Verification items for the finished model (mm, model axes). Face numbers are marked on the shaded views. Give positions to 0.01 mm unless a question says otherwise; leave off trailing zeros. Loops run counter-clockwise (first coordinate to the right, second up) from the corner with the lowest first, then second, coordinate; pieces in that order, holes last. Notation, with made-up numbers: (23, 12) - (70, 12) arc R28 cw to (70, 49) - close; hole circle Ø1 at (52, 66). An arc over 180 degrees is marked (long way). Use one line per item in the form item = value.
```python
from build123d import *

# Parameters (mm, degrees)
SKETCH_1_W      = 134
SKETCH_1_H      = 90
EXTRUDE_1_DEPTH = 5
EXTRUDE_2_DEPTH = 10
EXTRUDE_3_DEPTH = 8


with BuildPart() as part:
    # Эскиз1 → Бобышка-Вытянуть1 (new body)
    with BuildSketch(Plane(origin=(0, 0, 0), x_dir=(1, 0, 0), z_dir=(0, 1, 0))):
        Rectangle(SKETCH_1_W, SKETCH_1_H)
    extrude(amount=EXTRUDE_1_DEPTH)

    # Эскиз2 → Бобышка-Вытянуть2 (add)
    with BuildSketch(Plane(origin=(0, 5, 0), x_dir=(1, 0, 0), z_dir=(0, 1, 0))):
        Polygon((-51.5, -45), (-47, -45), (-47, -25), (-52, -25), (-52, 30), (52, 30), (52, -25), (42, -25), (42, -45), (51.5, -45), (67, -45), (67, -25), (67, 30), (67, 45), (51.5, 45), (-51.5, 45), (-67, 45), (-67, 30), (-67, -25), (-67, -45), align=None)
    extrude(amount=EXTRUDE_2_DEPTH)

    # Эскиз3 → Бобышка-Вытянуть3 (add)
    with BuildSketch(Plane(origin=(0, 15, 0), x_dir=(1, 0, 0), z_dir=(0, 1, 0))):
        Polygon((62, -45), (67, -45), (67, 40), (67, 45), (61.5, 45), (-61.5, 45), (-67, 45), (-67, 40), (-67, -45), (-62, -45), (-62, 40), (62, 40), align=None)
    extrude(amount=EXTRUDE_3_DEPTH)


solid = part.part
```
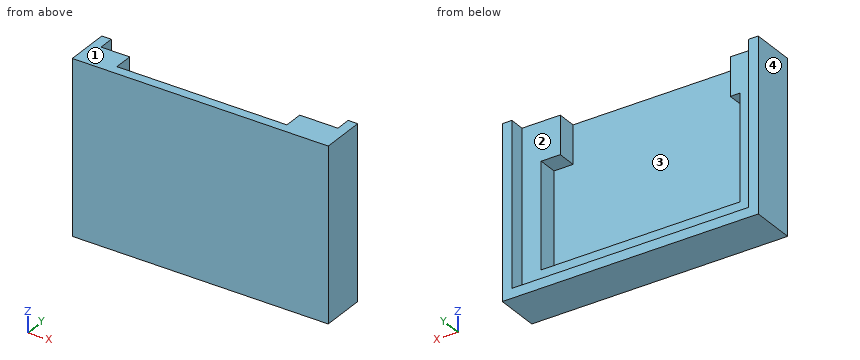
1. Scan lines: probe 1 along X at (y, z) = (8.5, 17); probe 2 along X at (y, z) = (16, -5.5); probe 3 along Z at (x, y) = (51, 13). Record each from-to range of solid material in increasing order.
Result set:
probe_1 = -67 to -52, 52 to 67
probe_2 = -67 to -62, 62 to 67
probe_3 = -45 to -30, 25 to 45
2. Section check A-A, the plane y = 20. Record the cut outline in (x, z).
Result set:
outline = (-67, -45) - (67, -45) - (67, 45) - (62, 45) - (62, -40) - (-62, -40) - (-62, 45) - (-67, 45) - close
3. Section check B-B, the plane z = -11.5. Record the cut outline in (x, y), then the cut area to 3 significant figures.
Result set:
outline = (-67, 0) - (67, 0) - (67, 23) - (62, 23) - (62, 15) - (52, 15) - (52, 5) - (-52, 5) - (-52, 15) - (-62, 15) - (-62, 23) - (-67, 23) - close
area = 1,050 mm²
4. Depth check by flat-ended pin: pin 1 Ø6 at (x, y) = (-4, 6.5) entering from +Z; pin 2 Ø10 at (x, z) = (18, -31.5) entering from +Y; pin 3 Ø5 at (x, y) = (25.5, 16.5) entering from +Z; pin 4 Ø6.5 at (x, y) = (22.5, 18.5) entering from +Z. Enter the tip coordinate at first touch or a pass-through.
Result set:
pin_1 = 45
pin_2 = 15
pin_3 = -30
pin_4 = -40
5. Section check C-C, the plane x = 48. Record the cut outline in (y, z).
Result set:
outline = (0, -45) - (23, -45) - (23, -40) - (15, -40) - (15, -30) - (5, -30) - (5, 25) - (15, 25) - (15, 45) - (0, 45) - close
6. Draft check along X on the marked faces 1, 2, 3 and 4. Enter one of: released by +X, released by -X, zero draft, split by the parting line, or undercut.
Result set:
face_1 = zero draft
face_2 = undercut
face_3 = undercut
face_4 = released by -X
7. Section check D-D, the plane y = 11. Record the cut outline in (x, z).
Result set:
outline = (-67, -45) - (67, -45) - (67, 45) - (42, 45) - (42, 25) - (52, 25) - (52, -30) - (-52, -30) - (-52, 25) - (-47, 25) - (-47, 45) - (-67, 45) - close
